Can you work these out from the model? Positions are in its coordinate system, mm. Face numbers are marked on the shaded views. A direction names the side the tool comes from. Give positions to 0.01 mm unless a question says otherwise; leave off trailing zeros. Return JSON: item names as keys, results as strings.
```python
from build123d import *

# Parameters (mm, degrees)
F0_W      = 127
F0_H      = 101.6
F1_DEPTH  = 25.4
F2_W      = 101.6
F2_H      = 76.2
F3_DEPTH  = 50.8
F3_TAPER  = -12
F4_R      = 31.75
F5_DEPTH  = 12.7
F6_R      = 20.9296
F7_DEPTH  = 12.7
F8_R      = 3.175
F9_DEPTH  = 76.201
F11_DEPTH = 12.7


with BuildPart() as f1:
    # F0 (on Top) → F1 (new body)
    with BuildSketch(Plane.XY):
        Rectangle(F0_W, F0_H)
    extrude(amount=F1_DEPTH)

    # F2 (on face) → F3 (join)
    with BuildSketch(Plane.XY.offset(25.4)):
        Rectangle(F2_W, F2_H)
    extrude(amount=F3_DEPTH, taper=F3_TAPER)

    # F4 (on face) → F5 (cut)
    with BuildSketch(Plane.XY.offset(76.2)):
        Circle(F4_R)
    extrude(amount=-F5_DEPTH, mode=Mode.SUBTRACT)

    # F6 (on face) → F7 (join)
    with BuildSketch(Plane.XY.offset(63.5)):
        Circle(F6_R)
    extrude(amount=F7_DEPTH)

    # F8 (on face) → F9 (cut, through all)
    with BuildSketch(Plane.XY.offset(76.2)):
        with Locations((-38.1, 0)):
            Circle(F8_R)
        with Locations((0, 39.6875)):
            Circle(F8_R)
    extrude(amount=-F9_DEPTH, mode=Mode.SUBTRACT)

    # F10 (on face) → F11 (cut)
    with BuildSketch(Plane.XY.offset(76.2)):
        with BuildLine():
            ThreePointArc((19.991276409, -6.1965332), (20.9296, 0), (19.991276409, 6.1965332))
            Line((19.991276409, 6.1965332), (-19.991276409, 6.1965332))
            ThreePointArc((-19.991276409, 6.1965332), (-20.9296, 0), (-19.991276409, -6.1965332))
            Line((-19.991276409, -6.1965332), (19.991276409, -6.1965332))
        make_face()
    extrude(amount=-F11_DEPTH, mode=Mode.SUBTRACT)


solid = f1.part
```
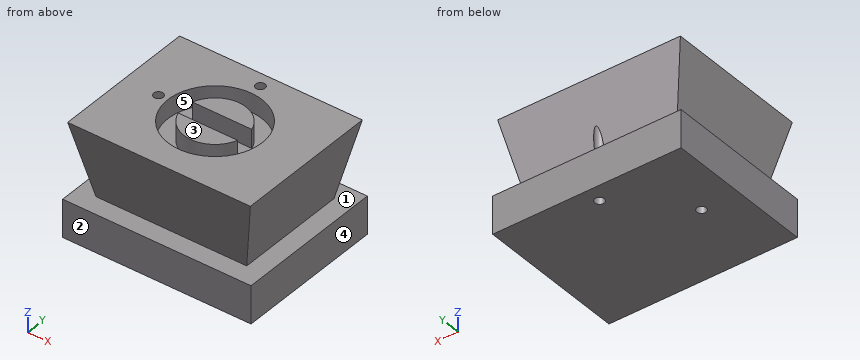
1. If I drill on L1, parallel to Y at x = 9, z = 64; L2, parallel to X at y = 16, z = 66; L3, parallel to Y at x = -8, z = 64, over which ranges is the centre line in solid material (lowest first)? Write a range as [from, to].
Checks:
{"L1": "[-46.3, -30.45], [-18.9, -6.2], [6.2, 18.9], [30.45, 46.3]", "L2": "[-59.43, -27.42], [-13.49, 13.49], [27.42, 59.43]", "L3": "[-46.3, -30.73], [-19.34, -6.2], [6.2, 19.34], [30.73, 46.3]"}
2. Thinking about a two-plate mould opening in X: for the marked faces 3, 4 and 5, which applies, +X half, -X half, draft (parallel to the pull), parting line (faces both ways), or undercut?
Checks:
{"face 3": "draft", "face 4": "+X half", "face 5": "undercut"}
3. For pin 1 Ø1 at (y, z) = (-5.5, 30) entering from -X; pin 2 Ø4 at (x, y) = (0, 39.69) entering from -Z; pin 3 Ø10 at (x, z) = (5.5, 71.5) entering from +Y; pin 4 Ø8 at (y, z) = (33.5, 33) entering from -X, each with a flat end and sliding along its axis, tell me the tip position at first contact or that it passes through.
Checks:
{"pin 1": "x = -51.88", "pin 2": "through", "pin 3": "y = 48.9", "pin 4": "x = -53.27"}
4. On a 3-axis mill with a long thin cutter (end or side, diameter ignored), from which of +Z, -Z, +X, -X, +Y, -Y can I reach the whole of each face in a straight line? I mean the marked faces 1 and 2. Say none if no direction works.
Checks:
{"face 1": "none", "face 2": "+Z, -Z, +X, -X, -Y"}
5. Suppose I cut it at A-A (x = 0). State how many separate pieces and enclosed holes the cut face has, plus the area to 3 significant figures.
Checks:
{"separate pieces": "3", "enclosed holes": "0", "area": "6,140 mm^2"}
